Verification items for the finished model (mm, model axes). Face numbers are marked on the shaded views. A direction names the side the tool comes from. Coordinates: 2 decimals unless noted, no trailing zeros. Order: outer loops, then holes, each group sorted by start corner. A loop starts at its lowest first (then second) coordinate and runs counter-clockwise, first axis right, second up. Notation, with made-up numbers: (-23, 88.25) -> (32, 88.25) arc R19 cw to (32, 118.25) -> close; hole circle Ø8 at (75.5, -24). An arc over 180 degrees is marked (long way). Write item = value, one per line. Start each with the question number.
1. Cross-section at A-A on y = 9. Record the cut outline in (x, z) (3 decimals).
2. Go/stop test with flat-tipped pins: P1, Ø4.5, axis at x = 65.73, z = -7.62, coming from the -Y side; P2, Ø4, axis at x = 76.2, y = 25.4, coming from the -Z side (3 decimals); P3, Ø8, axis at x = -50, z = 49.5, coming from the +Y side (3 decimals). Record where each tip stops, or that it passes through.
3. Cross-section at B-B on z = 12.7. Record the cut outline in (x, y) (1 decimal).
4. Set-up check for the marked faces 4 and 5: record each of +Z, -Z, +X, -X, +Y, -Y from which the full face is reachable in a straight line by a thin tool's end or side.
5. Thickness scan on line 1 along X through (y, z) = (1.9, -7.62); line 2 along Z through (x, y) = (-80.5, 10.5) (3 decimals); line 3 along X through (y, z) = (1.85, -43.18). Record the ranges inside material, lowest first. Write a range as from..to.
6. Cross-section at D-D on x = 25. Record the cut outline in (y, z) (3 decimals).
7. Cross-section at C-C on z = -43.18. Record the cut outline in (x, y) (3 decimals).
8. Release check for a two-part mould opening along Z. For the marked faces 1, 2 and 3 record: +Z half, -Z half, draft (parallel to the pull), parting line (faces both ways), or undercut.
from build123d import *

# Parameters (mm, degrees)
SKETCH1_W           = 177.8
SKETCH1_H           = 127
BOSS_EXTRUDE1_DEPTH = 3.175
EDGE_FLANGE1_DEPTH  = 177.8
EDGE_FLANGE2_DEPTH  = 177.8
SKETCH17_R          = 2.54
CUT_EXTRUDE1_DEPTH  = 5.08
FILLET1_R           = 12.7
SKETCH18_R          = 3.175
CUT_EXTRUDE2_DEPTH  = 5.08
SKETCH19_R          = 14.2875
CUT_EXTRUDE3_DEPTH  = 12.7
SKETCH20_R          = 9.525
CUT_EXTRUDE4_DEPTH  = 12.7
SKETCH21_R          = 2.54
CUT_EXTRUDE6_DEPTH  = 12.7


# Sheet-metal steps are written as plain solids
with BuildPart() as part:
    # Sketch1 → Boss-Extrude1 (new body)
    with BuildSketch(Plane(origin=(0, 0, 0), x_dir=(1, 0, 0), z_dir=(0, 1, 0))):
        Rectangle(SKETCH1_W, SKETCH1_H)
    extrude(amount=BOSS_EXTRUDE1_DEPTH)

    # Edge-Flange1 section (across the edge) → Edge-Flange1 (add)
    with BuildSketch(Plane(origin=(88.9, 3.175, -66.675), x_dir=(0, 0, 1), z_dir=(-1, 0, 0))):
        with BuildLine():
            Line((-3.175, 3.175), (-3.175, 34.925))
            Line((-3.175, 34.925), (0, 34.925))
            Line((0, 34.925), (0, 3.175))
            ThreePointArc((0, 3.175), (0.92993597, 0.92993597), (3.175, 0))
            Line((3.175, 0), (3.175, -3.175))
            ThreePointArc((3.175, -3.175), (-1.315128061, -1.315128061), (-3.175, 3.175))
        make_face()
    extrude(amount=EDGE_FLANGE1_DEPTH)

    # Edge-Flange2 section (across the edge) → Edge-Flange2 (add)
    with BuildSketch(Plane(origin=(-88.9, 3.175, 66.675), x_dir=(0, 0, -1), z_dir=(1, 0, 0))):
        with BuildLine():
            Line((-3.175, 3.175), (-3.175, 34.925))
            Line((-3.175, 34.925), (0, 34.925))
            Line((0, 34.925), (0, 3.175))
            ThreePointArc((0, 3.175), (0.92993597, 0.92993597), (3.175, 0))
            Line((3.175, 0), (3.175, -3.175))
            ThreePointArc((3.175, -3.175), (-1.315128061, -1.315128061), (-3.175, 3.175))
        make_face()
    extrude(amount=EDGE_FLANGE2_DEPTH)

    # Sketch17 → Cut-Extrude1 (cut)
    with BuildSketch(Plane(origin=(0, 0, -69.85), x_dir=(-1, 0, 0), z_dir=(0, 0, -1))):
        with Locations(Location((-76.2, 25.4, 0), (0, 0, 90))):
            Circle(SKETCH17_R)
        with Locations(Location((-54.428571429, 25.4, 0), (0, 0, 90))):
            Circle(SKETCH17_R)
        with Locations(Location((-32.657142857, 25.4, 0), (0, 0, 90))):
            Circle(SKETCH17_R)
        with Locations(Location((-10.885714286, 25.4, 0), (0, 0, 90))):
            Circle(SKETCH17_R)
        with Locations(Location((10.885714286, 25.4, 0), (0, 0, 90))):
            Circle(SKETCH17_R)
        with Locations(Location((32.657142857, 25.4, 0), (0, 0, 90))):
            Circle(SKETCH17_R)
        with Locations(Location((54.428571429, 25.4, 0), (0, 0, 90))):
            Circle(SKETCH17_R)
        with Locations(Location((76.2, 25.4, 0), (0, 0, 90))):
            Circle(SKETCH17_R)
    extrude(amount=-CUT_EXTRUDE1_DEPTH, mode=Mode.SUBTRACT)

    # Fillet1
    fillet1_edges = [part.edges().sort_by_distance(p)[0] for p in [
        (88.9, 38.1, -68.2625),
        (-88.9, 38.1, -68.2625),
        (-88.9, 38.1, 68.2625),
        (88.9, 38.1, 68.2625),
    ]]
    fillet(fillet1_edges, radius=FILLET1_R)

    # Sketch18 → Cut-Extrude2 (cut)
    with BuildSketch(Plane(origin=(0, 0, 66.675), x_dir=(-1, 0, 0), z_dir=(0, 0, -1))):
        with Locations((69.85, 25.4)):
            Circle(SKETCH18_R)
        with Locations((-69.85, 25.4)):
            Circle(SKETCH18_R)
    extrude(amount=-CUT_EXTRUDE2_DEPTH, mode=Mode.SUBTRACT)

    # Sketch19 → Cut-Extrude3 (cut)
    with BuildSketch(Plane(origin=(0, 0, 0), x_dir=(-1, 0, 0), z_dir=(0, -1, 0))):
        with Locations(Location((0, -12.7, 0), (0, 0, 90))):
            Circle(SKETCH19_R)
    extrude(amount=-CUT_EXTRUDE3_DEPTH, mode=Mode.SUBTRACT)

    # Sketch20 → Cut-Extrude4 (cut)
    with BuildSketch(Plane.XZ):
        with Locations(Location((47.586884748, -25.4, 0), (0, 0, 270))):
            Circle(SKETCH20_R)
        with Locations(Location((-47.586884748, -25.4, 0), (0, 0, 270))):
            Circle(SKETCH20_R)
    extrude(amount=-CUT_EXTRUDE4_DEPTH, mode=Mode.SUBTRACT)

    # Sketch21 → Cut-Extrude6 (cut)
    with BuildSketch(Plane(origin=(0, 0, 0), x_dir=(-1, 0, 0), z_dir=(0, -1, 0))):
        with Locations(Location((-65.726112956, 7.62, 0), (0, 0, 90))):
            Circle(SKETCH21_R)
        with Locations(Location((-29.447656539, 43.18, 0), (0, 0, 90))):
            Circle(SKETCH21_R)
        with Locations(Location((65.726112956, 7.62, 0), (0, 0, 90))):
            Circle(SKETCH21_R)
        with Locations(Location((29.447656539, 43.18, 0), (0, 0, 90))):
            Circle(SKETCH21_R)
    extrude(amount=-CUT_EXTRUDE6_DEPTH, mode=Mode.SUBTRACT)


solid = part.part
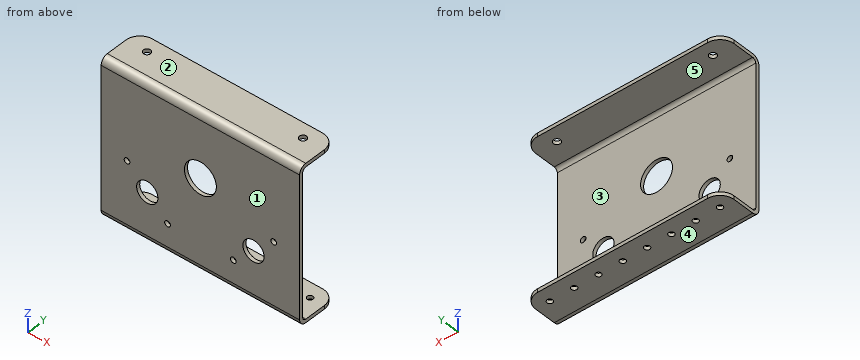
Worked out:
q1.outline = (-88.9, -69.85) -> (88.9, -69.85) -> (88.9, -66.675) -> (-88.9, -66.675) -> close; (-88.9, 66.675) -> (88.9, 66.675) -> (88.9, 69.85) -> (-88.9, 69.85) -> close
q2.P1 = through
q2.P2 = 66.675
q2.P3 = 3.175
q3.outline = (-88.9, 0) -> (-14.3, 0) -> (-14.3, 3.2) -> (-88.9, 3.2) -> close; (14.3, 0) -> (88.9, 0) -> (88.9, 3.2) -> (14.3, 3.2) -> close
q4.face_4 = -Z, +X, -X, +Y, -Y
q4.face_5 = +X, -X, +Y
q5.line_1 = -88.9..-68.27, -63.19..63.19, 68.27..88.9
q5.line_2 = -69.85..-66.675, 66.675..69.85
q5.line_3 = -88.9..-31.99, -26.91..26.91, 31.99..88.9
q6.outline = (0, -63.5) arc R6.35 ccw to (6.35, -69.85) -> (38.1, -69.85) -> (38.1, -66.675) -> (6.35, -66.675) arc R3.175 cw to (3.175, -63.5) -> (3.175, 63.5) arc R3.175 cw to (6.35, 66.675) -> (38.1, 66.675) -> (38.1, 69.85) -> (6.35, 69.85) arc R6.35 ccw to (0, 63.5) -> close
q7.outline = (-88.9, 0) -> (-31.988, 0) -> (-31.988, 3.175) -> (-88.9, 3.175) -> close; (-26.908, 0) -> (26.908, 0) -> (26.908, 3.175) -> (-26.908, 3.175) -> close; (31.988, 0) -> (88.9, 0) -> (88.9, 3.175) -> (31.988, 3.175) -> close
q8.face_1 = draft
q8.face_2 = +Z half
q8.face_3 = undercut
